Autodesk Fusion 360 part; units mm, degrees
sketch "Sketch1" plane through (0, 0, 0) normal (0, 0, 1) x (1, 0, 0)
  line L0 (0, 0) -> (0, 75)
  line L1 (0, 75) -> (75, 75)
  line L2 (75, 75) -> (75, 0)
  line L3 (75, 0) -> (0, 0)
  line L4 (-5, -5) -> (-5, 80)
  line L5 (-5, 80) -> (80, 80)
  line L6 (80, 80) -> (80, -5)
  line L7 (80, -5) -> (-5, -5)
  dimension "d1" = 75
  dimension "d2" = 75
  dimension "d3" = 75
  dimension "d4" = 75
  dimension "d5" = 85
  dimension "d6" = 85
  dimension "d7" = 85
  dimension "d8" = 85
extrude "Extrude1" add sketch "Sketch1" along normal blind 10
sketch "Sketch2" plane through (0, 0, 0) normal (0, 1, 0) x (1, 0, 0)
sketch "Sketch3" plane through (0, 0, 0) normal (0, 0, 1) x (1, 0, 0)
  line L0 (0, 0) -> (75, 0)
  line L1 (75, 0) -> (75, 75)
  line L2 (75, 75) -> (0, 75)
  line L3 (0, 75) -> (0, 0)
extrude "Extrude2" add sketch "Sketch3" along normal blind 4
sketch "Sketch4" plane through (0, 0, 4) normal (0, 0, 1) x (-1, 0, 0)
  line L0 (0, -75) -> (0, 0)
  line L1 (0, 0) -> (-75, 0)
  line L2 (-75, 0) -> (-75, -75)
  line L3 (-75, -75) -> (0, -75)
  line L4 (0, 0) -> (-75, -75)
  line L5 (-75, 0) -> (0, -75)
  line L6 (-37.5, -37.5) -> (-37.5, -65)
  line L7 (-37.5, -37.5) -> (-65, -37.5)
  line L8 (-65, -37.5) -> (-65, -10)
  line L9 (-37.5, -65) -> (-10, -65)
  line L10 (-10, -65) -> (-65, -65)
  line L11 (-65, -65) -> (-65, -10)
  line L12 (-65, -10) -> (-10, -10)
  line L13 (-10, -10) -> (-10, -65)
  line L14 (-65, -65) -> (-60, -65)
  line L15 (-60, -65) -> (-60, -60)
  circle A0 centre (-60, -60) radius 1.625
  line L16 (-10, -10) -> (-10, -27.5)
  line L17 (-10, -27.5) -> (-15, -27.5)
  circle A1 centre (-15, -27.5) radius 1.625
  dimension "d13" = 27.5
  dimension "d14" = 27.5
  dimension "d15" = 27.5
  dimension "d16" = 27.5
  dimension "d17" = 5
  dimension "d18" = 5
  dimension "d19" = 3.25
  dimension "d20" = 17.5
  dimension "d21" = 5
  dimension "d22" = 3.25
extrude "Extrude3" add sketch "Sketch4" along normal blind 3 draft -4 contours A1 | L4 A0 | L4 L15 A0 | L4 L15 A0
sketch "Sketch5" plane through (0, 0, 10) normal (0, 0, 1) x (-1, 0, 0)
  line L0 (-75, -75) -> (-75, 0)
  line L1 (-75, 0) -> (0, 0)
  line L2 (0, 0) -> (0, -75)
  line L3 (0, -75) -> (-75, -75)
  line L4 (-80, 5) -> (-80, -80)
  line L5 (-80, -80) -> (5, -80)
  line L6 (5, -80) -> (5, 5)
  line L7 (5, 5) -> (-80, 5)
  line L8 (5, 5) -> (0, 0)
  line L9 (5, 0) -> (0, 5)
  circle A0 centre (2.5, 2.5) radius 1.5
  line L10 (-75, -75) -> (-80, -80)
  line L11 (-80, -75) -> (-75, -80)
  circle A1 centre (-77.5, -77.5) radius 1.5
  line L12 (0, -75) -> (5, -80)
  line L13 (5, -75) -> (0, -80)
  circle A2 centre (2.5, -77.5) radius 1.5
  line L14 (-80, 5) -> (-75, 0)
  line L15 (-75, 5) -> (-80, 0)
  circle A3 centre (-77.5, 2.5) radius 1.5
  dimension "d25" = 3
  dimension "d26" = 3
  dimension "d27" = 3
  dimension "d28" = 3
extrude "Extrude4" add sketch "Sketch5" along normal blind 4 draft -3 contours L10 L11 A1 | L10 L11 A1 | L14 L15 A3 | L14 L15 A3 | L12 L13 A2 | L12 L13 A2 | L10 L11 A1 | L10 L11 A1 | L8 L9 A0 | L8 L9 A0 | L14 L15 A3 | L14 L15 A3 | L12 L13 A2 | L12 L13 A2 | L8 L9 A0 | L8 L9 A0
sketch "Sketch6" plane through (0, 0, 7) normal (0, 0, 1) x (-1, 0, 0)
  circle A0 centre (-60, -60) radius 1.4152
equation "d13 = ( 55 / 2 ) * 1 mm"
equation "d14 = ( 55 / 2 ) * 1 mm"
equation "d15 = ( 55 / 2 ) * 1 mm"
equation "d16 = ( 55 / 2 ) * 1 mm"
Geometry: final body of the model. Coordinates: model frame, mm. A direction names the side the tool comes from. Give positions to 0.01 mm unless a question says otherwise; leave off trailing zeros. Order: outer loops, then holes, each group sorted by start corner. A loop starts at its lowest first (then second) coordinate and runs counter-clockwise, first axis right, second up. Notation, with made-up numbers: (24.25, -40) -> (59.25, -40) arc R17 ccw to (59.25, -14) -> close; hole circle Ø4 at (88.5, 80). An arc over 180 degrees is marked (long way). Put each result on its own line as item: value.
Q1. Section B-B, the plane x = 5. Return loops of the section in (y, z), then the cut area to 3 significant figures.
Here are the results:
outline: (-5, 0) -> (80, 0) -> (80, 10) -> (75, 10) -> (75, 4) -> (0, 4) -> (0, 10) -> (-5, 10) -> close
area: 400 mm^2
Q2. Material intervals for L1, parallel to Y at x = 49, z = 7.5; L2, parallel to Z at x = 28, y = 13, sorted ascending.
Here are the results:
L1: y = -5 to 0, 75 to 80
L2: z = 0 to 4
Q3. Draft query along Y for faces 3 (the face through (-2.515, 78.897, 11.972)), 4 (the face through (-2.515, -1.103, 11.972)), 5 (the face through (37, 38, 0)). Return one class per face: released by +Y, released by -Y, zero draft, split by the parting line, or undercut.
Here are the results:
face 3: released by +Y
face 4: undercut
face 5: zero draft
Q4. Section A-A, the plane z = 8.5. Return loops of the section in (x, y).
Here are the results:
outline: (-5, -5) -> (80, -5) -> (80, 80) -> (-5, 80) -> close; hole (0, 0) -> (75, 0) -> (75, 75) -> (0, 75) -> close
Q5. Pin query (flat end, axial travel): pin 1 (0.7 mm diameter, centred on x = 60.5, y = 60, fed in from +Z); pin 2 (3 mm diameter, centred on x = 29, y = 49, fed in from +Z). Return the tip coordinate at first contact, or that it passes through.
Here are the results:
pin 1: stops at z = 7
pin 2: stops at z = 4
Q6. Reachability of faces 1 (the face through (37, 80, 5)), 2 (the face through (15, 27, 7)) from +Z, -Z, +X, -X, +Y, -Y: full face, straight path, thin tool, end or side. Return the list, or none.
Here are the results:
face 1: +Z, -Z, +X, -X, +Y
face 2: +Z
Q7. Section D-D, the plane y = 27.5. Return loops of the section in (x, z) (3 decimals), then the cut area to 3 significant figures.
Here are the results:
outline: (-5, 0) -> (80, 0) -> (80, 10) -> (75, 10) -> (75, 4) -> (16.625, 4) -> (16.415, 7) -> (13.585, 7) -> (13.375, 4) -> (0, 4) -> (0, 10) -> (-5, 10) -> close
area: 409 mm^2
